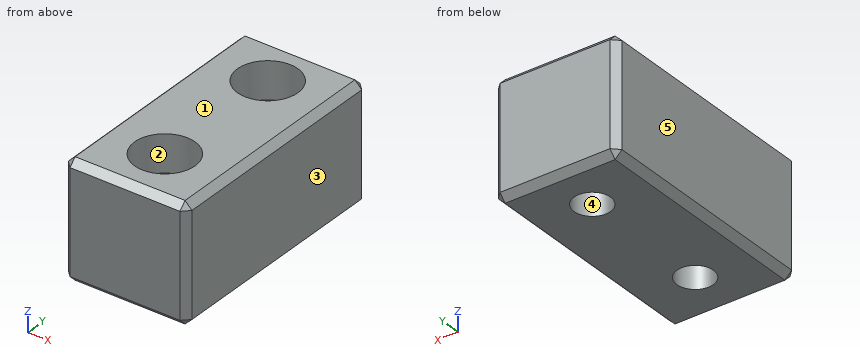
```python
from build123d import *

# Parameters (mm, degrees)
SKETCH076_W         = 18
SKETCH076_H         = 35
PAD038_DEPTH        = 17
HOLE008_D           = 5.3
HOLE008_DEPTH       = 25
HOLE008_CBORE_D     = 8.8
HOLE008_CBORE_DEPTH = 5.4
CHAMFER021_SIZE     = 1


with BuildPart() as part:
    # Sketch076 → Pad038 (new body)
    with BuildSketch(Plane.XY.offset(-51)):
        with Locations((101, 222.5)):
            Rectangle(SKETCH076_W, SKETCH076_H)
    extrude(amount=PAD038_DEPTH)

    # Hole008
    with Locations(Plane.XY.offset(-34)):
        with Locations((101, 232.75), (101, 212.75)):
            CounterBoreHole(HOLE008_D / 2, HOLE008_CBORE_D / 2, HOLE008_CBORE_DEPTH, depth=HOLE008_DEPTH)

    # Chamfer021
    chamfer021_edges = [part.edges().sort_by_distance(p)[0] for p in [
        (92, 240, -42.5),
        (110, 240, -42.5),
        (101, 240, -51),
        (101, 240, -34),
        (110, 205, -42.5),
        (110, 222.5, -51),
        (110, 222.5, -34),
        (92, 205, -42.5),
        (92, 222.5, -51),
        (92, 222.5, -34),
        (101, 205, -51),
        (101, 205, -34),
    ]]
    chamfer(chamfer021_edges, length=CHAMFER021_SIZE)


with BuildPart() as part_1:
    # Body001010 placement: moved
    add(part.part.moved(Location((0, 3.75, 0))))


solid = part_1.part
```
Input: part model. Units: mm. Frame: model coordinates. Face numbers are marked on the shaded views. A direction names the side the tool comes from. Coordinates: 2 decimals unless noted, no trailing zeros. Write each loop counter-clockwise with the first axis right and the second up, starting at its lowest first coordinate (ties: lowest second). Pieces come first, ordered by that corner, then holes.
1) Set-up query: the marked faces 1 and 2. Return all of +Z, -Z, +X, -X, +Y, -Y with unobstructed straight access to the full face (end or side cutting, diameter ignored); none if empty.
2) Section B-B on x = 101. Output: boundary loops of the cut face in (y, z).
3) Section C-C on z = -49. Output: boundary loops of the cut face in (x, y).
4) Mould query, pull axis X, two halves, no side actions, for the marked faces 3, 4 and 5. Classes: pulls with the +X half, pulls with the -X half, needs draft (parallel to the pull), parting line crosses it, or undercut.
5) Material intervals for line 1 along Y through (x, z) = (101, -36.35); line 2 along Y through (x, z) = (101, -43); line 3 along X through (y, z) = (218, -42), sorted ascending.
6) Pin query (flat end, axial travel): pin 1 Ø8.5 at (x, y) = (101, 236.5) entering from +Z; pin 2 Ø4 at (x, y) = (101, 216.5) entering from +Z. Return the tip coordinate at first contact, or that it passes through.
7) Section D-D on y = 233. Output: boundary loops of the cut face in (x, z), and give its area (3 significant figures).
8) Section A-A on y = 216.5. Output: boundary loops of the cut face in (x, z), and give its area (3 significant figures).
Check result:
1. face 1: +Z, +X, -X, +Y, -Y
1. face 2: +Z
2. outline: (208.75, -50) - (209.75, -51) - (213.85, -51) - (213.85, -39.4) - (212.1, -39.4) - (212.1, -34) - (209.75, -34) - (208.75, -35) - close; (219.15, -51) - (233.85, -51) - (233.85, -39.4) - (232.1, -39.4) - (232.1, -34) - (220.9, -34) - (220.9, -39.4) - (219.15, -39.4) - close; (239.15, -51) - (242.75, -51) - (243.75, -50) - (243.75, -35) - (242.75, -34) - (240.9, -34) - (240.9, -39.4) - (239.15, -39.4) - close
3. outline: (92, 209.75) - (93, 208.75) - (109, 208.75) - (110, 209.75) - (110, 242.75) - (109, 243.75) - (93, 243.75) - (92, 242.75) - close; hole circle Ø5.3 at (101, 216.5); hole circle Ø5.3 at (101, 236.5)
4. face 3: pulls with the +X half
4. face 4: undercut
4. face 5: pulls with the -X half
5. line 1: y = 208.75 to 212.1, 220.9 to 232.1, 240.9 to 243.75
5. line 2: y = 208.75 to 213.85, 219.15 to 233.85, 239.15 to 243.75
5. line 3: x = 92 to 98.82, 103.18 to 110
6. pin 1: stops at z = -39.4
6. pin 2: passes through
7. outline: (92, -50) - (93, -51) - (109, -51) - (110, -50) - (110, -35) - (109, -34) - (103.67, -34) - (103.67, -39.4) - (98.33, -39.4) - (98.33, -34) - (93, -34) - (92, -35) - close
7. area: 275 mm2
8. outline: (92, -50) - (93, -51) - (98.35, -51) - (98.35, -39.4) - (96.6, -39.4) - (96.6, -34) - (93, -34) - (92, -35) - close; (103.65, -51) - (109, -51) - (110, -50) - (110, -35) - (109, -34) - (105.4, -34) - (105.4, -39.4) - (103.65, -39.4) - close
8. area: 195 mm2
